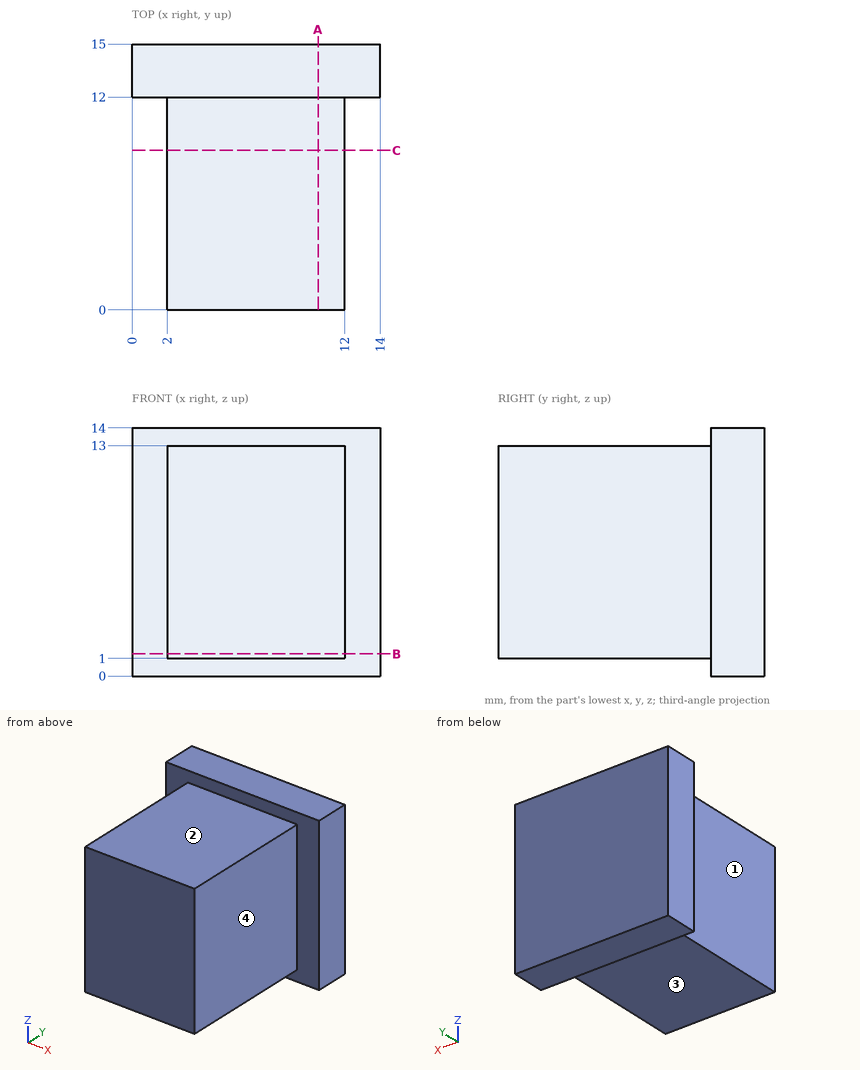
Part print with two shaded views. Sizes in mm from the minimum x, y, z corner. A direction names the side the tool comes from. Coordinates: 2 decimals unless noted, no trailing zeros. Write each loop counter-clockwise with the first axis right and the second up, starting at its lowest first coordinate (ties: lowest second). Pieces come first, ordered by that corner, then holes.
1. Drop flat-ended pins along their axis: pin 1 (5 mm diameter, centred on x = 6.5, z = 1.5, fed in from -Y); pin 2 (5 mm diameter, centred on y = 6, z = 5.5, fed in from +X); pin 3 (1.5 mm diameter, centred on x = 1.5, y = 5.5, fed in from -Z); pin 4 (1 mm diameter, centred on x = 4.5, y = 3.5, fed in from +Z). Give the stop position or say it passes through.
Answer block:
pin 1: stops at y = 0
pin 2: stops at x = 12
pin 3: stops at z = 1
pin 4: stops at z = 13
2. Band-saw the part on A-A, the plane x = 10.5. Give the cut face in (y, z), and give its area (3 significant figures).
Answer block:
outline: (0, 1) - (12, 1) - (12, 0) - (15, 0) - (15, 14) - (12, 14) - (12, 13) - (0, 13) - close
area: 186 mm2
3. 3-axis set-ups, long thin cutter, end or side, ignore diameter. For the marked faces 1, 2, 3 and 4: which of +Z, -Z, +X, -X, +Y, -Y reach the whole face in a straight line?
Answer block:
face 1: +Z, -Z, -X, -Y
face 2: +Z, +X, -X, -Y
face 3: -Z, +X, -X, -Y
face 4: +Z, -Z, +X, -Y
4. Band-saw the part on C-C, the plane y = 9. Give the cut face in (x, z), and give its area (3 significant figures).
Answer block:
outline: (2, 1) - (12, 1) - (12, 13) - (2, 13) - close
area: 120 mm2
5. Band-saw the part on B-B, the plane z = 1.25. Give the cut face in (x, y), and give its area (3 significant figures).
Answer block:
outline: (0, 12) - (2, 12) - (2, 0) - (12, 0) - (12, 12) - (14, 12) - (14, 15) - (0, 15) - close
area: 162 mm2
6. Drill centre lines: probe 1 along Y at (x, z) = (12.5, 3.75); probe 2 along X at (y, z) = (2.5, 9.5); probe 3 along Z at (x, y) = (2.25, 3.75). Where is each one in solid material? Low to high.
Answer block:
probe 1: y = 12 to 15
probe 2: x = 2 to 12
probe 3: z = 1 to 13
